Work out the finished part from the listing and answer in its coordinate system (mm). A direction names the side the tool comes from. Coordinates: 2 decimals unless noted, no trailing zeros. Loops run counter-clockwise (first coordinate to the right, second up) from the corner with the lowest first, then second, coordinate; pieces in that order, holes last. Notation, with made-up numbers: (-36, 38) - (-31, 38) arc R17 ccw to (-31, 52) - close; hole circle Ø11 at (75.5, -27.5). An arc over 180 degrees is marked (long way). Write each question's results on one line, items separated by ' | '. Start each with the question number.
1. A cutting plane is placed at C-C on z = -22. Determine the outline of the cut face in (x, y), then the cut area to 3 significant figures.
2. A cutting plane is placed at A-A on y = 20. Determine the outline of the cut face in (x, z), then the cut area to 3 significant figures.
3. Determine the mould class of faces 5 (the flat face through (32, 14, 110)), 6 (the flat face through (32, 13, -112)), 7 (the flat face through (100, 9, -111)), 8 (the flat face through (10, 1, -2)) for opening direction Z: released by +Z, released by -Z, zero draft, split by the parting line, or undercut.
4. Each of these flat-tipped pins is pushed along its axis until it touches: P1, Ø10, axis at y = 9, z = -52, coming from the +X side; P2, Ø0.6, axis at y = 13.5, z = -111, coming from the +X side; P3, Ø1, axis at x = 11, z = 111, coming from the +Y side; P4, Ø1.5, axis at x = 17.5, y = 24.5, coming from the +Z side. Where does it stop, or does it pass through?
5. Which of the six approach directions +Z, -Z, +X, -X, +Y, -Y give full straight-line access (tool end or side, diameter ignored) to faces 1 (the flat face through (-35, 9, -111)), 2 (the flat face through (32, 14, -110)), 3 (the flat face through (100, 8, 111)), 4 (the flat face through (-35, 9, 111))?
6. Find the intervals of material crossed by line 1 along Z through (x, y) = (-31.5, 7.5); line 2 along Y through (x, z) = (-22, -84); line 3 along X through (y, z) = (13, -18.5), in increasing order. Write a range as [from, to].
7. A cutting plane is placed at B-B on x = 15. Determine the outline of the cut face in (y, z).
from build123d import *

# Parameters (mm, degrees)
SKETCH1_W                    = 200
SKETCH1_H                    = 224
BOSS_EXTRUDE1_DEPTH          = 1
SKETCH41_W                   = 65
SKETCH41_H                   = 15
CUT_EXTRUDE2_DEPTH           = 40
EDGE_FLANGE1_STRIP_W         = 12
EDGE_FLANGE1_STRIP_H         = 2
EDGE_FLANGE1_STRIP_CUT_DEPTH = 135
EDGE_FLANGE1_DEPTH           = 135
SKETCH53_W                   = 194
SKETCH53_H                   = 2
BOSS_EXTRUDE2_DEPTH          = 20
CUT_EXTRUDE3_DEPTH           = 20
EDGE_FLANGE3_STRIP_W         = 12
EDGE_FLANGE3_STRIP_H         = 2
EDGE_FLANGE3_STRIP_CUT_DEPTH = 194
EDGE_FLANGE3_DEPTH           = 194
SKETCH58_W                   = 2
SKETCH58_H                   = 36
BOSS_EXTRUDE3_DEPTH          = 14
CUT_EXTRUDE4_DEPTH           = 10


# Sheet-metal steps are written as plain solids
with BuildPart() as part:
    # Sketch1 → Boss-Extrude1 (new, symmetric)
    with BuildSketch(Plane(origin=(0, 0, 0), x_dir=(1, 0, 0), z_dir=(0, 1, 0))):
        Rectangle(SKETCH1_W, SKETCH1_H)
    extrude(amount=BOSS_EXTRUDE1_DEPTH, both=True)

    # Sketch41 → Cut-Extrude2 (cut)
    with BuildSketch(Plane(origin=(0, 1, 0), x_dir=(1, 0, 0), z_dir=(0, 1, 0))):
        with Locations((-67.5, -104.5)):
            Rectangle(SKETCH41_W, SKETCH41_H)
        with Locations((-67.5, 104.5)):
            Rectangle(SKETCH41_W, SKETCH41_H)
    extrude(amount=-CUT_EXTRUDE2_DEPTH, mode=Mode.SUBTRACT)

    # Edge-Flange1 strip (across the edge) → Edge-Flange1 strip cut (cut)
    with BuildSketch(Plane(origin=(-35, 1, 112), x_dir=(0, 0, -1), z_dir=(1, 0, 0))):
        with Locations((-2, -1)):
            Rectangle(EDGE_FLANGE1_STRIP_W, EDGE_FLANGE1_STRIP_H)
    edge_flange1_strip_cut = extrude(amount=EDGE_FLANGE1_STRIP_CUT_DEPTH, mode=Mode.SUBTRACT)

    # Edge-Flange1 section (across the edge) → Edge-Flange1 (add)
    with BuildSketch(Plane(origin=(-35, 1, 112), x_dir=(0, 0, -1), z_dir=(1, 0, 0))):
        with BuildLine():
            Line((0, 2), (0, 23))
            Line((0, 23), (2, 23))
            Line((2, 23), (2, 2))
            ThreePointArc((2, 2), (2.585786438, 0.585786438), (4, 0))
            Line((4, 0), (4, -2))
            ThreePointArc((4, -2), (1.171572875, -0.828427125), (0, 2))
        make_face()
    edge_flange1 = extrude(amount=EDGE_FLANGE1_DEPTH)

    # Mirror1: Edge-Flange1 strip cut, Edge-Flange1 across plane
    add(edge_flange1_strip_cut.mirror(Plane.XY), mode=Mode.SUBTRACT)
    add(edge_flange1.mirror(Plane.XY))

    # Sketch53 → Boss-Extrude2 (add)
    with BuildSketch(Plane(origin=(100, 0, 0), x_dir=(0, 0, -1), z_dir=(1, 0, 0))):
        Rectangle(SKETCH53_W, SKETCH53_H)
    extrude(amount=BOSS_EXTRUDE2_DEPTH)

    # Sketch54 → Cut-Extrude3 (cut)
    with BuildSketch(Plane(origin=(0, 0, 110), x_dir=(-1, 0, 0), z_dir=(0, 0, -1))):
        with BuildLine():
            Line((-94.5, 8.506539698), (-94.5, 15.506539698))
            ThreePointArc((-94.5, 15.506539698), (-93, 17.006539698), (-91.5, 15.506539698))
            Line((-91.5, 15.506539698), (-91.5, 8.506539698))
            ThreePointArc((-91.5, 8.506539698), (-93, 7.006539698), (-94.5, 8.506539698))
        make_face()
        with BuildLine():
            Line((-85.5, 8.506539698), (-85.5, 15.506539698))
            ThreePointArc((-85.5, 15.506539698), (-84, 17.006539698), (-82.5, 15.506539698))
            Line((-82.5, 15.506539698), (-82.5, 8.506539698))
            ThreePointArc((-82.5, 8.506539698), (-84, 7.006539698), (-85.5, 8.506539698))
        make_face()
        with BuildLine():
            Line((-76.5, 8.506539698), (-76.5, 15.506539698))
            ThreePointArc((-76.5, 15.506539698), (-75, 17.006539698), (-73.5, 15.506539698))
            Line((-73.5, 15.506539698), (-73.5, 8.506539698))
            ThreePointArc((-73.5, 8.506539698), (-75, 7.006539698), (-76.5, 8.506539698))
        make_face()
        with BuildLine():
            Line((14.5, 8.506539698), (14.5, 15.506539698))
            ThreePointArc((14.5, 15.506539698), (16, 17.006539698), (17.5, 15.506539698))
            Line((17.5, 15.506539698), (17.5, 8.506539698))
            ThreePointArc((17.5, 8.506539698), (16, 7.006539698), (14.5, 8.506539698))
        make_face()
        with BuildLine():
            Line((5.5, 8.506539698), (5.5, 15.506539698))
            ThreePointArc((5.5, 15.506539698), (7, 17.006539698), (8.5, 15.506539698))
            Line((8.5, 15.506539698), (8.5, 8.506539698))
            ThreePointArc((8.5, 8.506539698), (7, 7.006539698), (5.5, 8.506539698))
        make_face()
        with BuildLine():
            Line((23.5, 8.506539698), (23.5, 15.506539698))
            ThreePointArc((23.5, 15.506539698), (25, 17.006539698), (26.5, 15.506539698))
            Line((26.5, 15.506539698), (26.5, 8.506539698))
            ThreePointArc((26.5, 8.506539698), (25, 7.006539698), (23.5, 8.506539698))
        make_face()
    cut_extrude3 = extrude(amount=-CUT_EXTRUDE3_DEPTH, mode=Mode.SUBTRACT)

    # Edge-Flange3 strip (across the edge) → Edge-Flange3 strip cut (cut)
    with BuildSketch(Plane(origin=(-100, 1, -97), x_dir=(1, 0, 0), z_dir=(0, 0, 1))):
        with Locations((-2, -1)):
            Rectangle(EDGE_FLANGE3_STRIP_W, EDGE_FLANGE3_STRIP_H)
    extrude(amount=EDGE_FLANGE3_STRIP_CUT_DEPTH, mode=Mode.SUBTRACT)

    # Edge-Flange3 section (across the edge) → Edge-Flange3 (add)
    with BuildSketch(Plane(origin=(-100, 1, -97), x_dir=(1, 0, 0), z_dir=(0, 0, 1))):
        with BuildLine():
            Line((0, 2), (0, 38))
            Line((0, 38), (2, 38))
            Line((2, 38), (2, 2))
            ThreePointArc((2, 2), (2.585786438, 0.585786438), (4, 0))
            Line((4, 0), (4, -2))
            ThreePointArc((4, -2), (1.171572875, -0.828427125), (0, 2))
        make_face()
    extrude(amount=EDGE_FLANGE3_DEPTH)

    # Sketch58 → Boss-Extrude3 (add)
    with BuildSketch(Plane.XY.offset(97)):
        with Locations((-99, 21)):
            Rectangle(SKETCH58_W, SKETCH58_H)
    boss_extrude3 = extrude(amount=BOSS_EXTRUDE3_DEPTH)

    # Mirror2: Cut-Extrude3, Boss-Extrude3 across plane
    add(cut_extrude3.mirror(Plane.XY), mode=Mode.SUBTRACT)
    add(boss_extrude3.mirror(Plane.XY))

    # Sketch59 → Cut-Extrude4 (cut)
    with BuildSketch(Plane(origin=(0, 1, 0), x_dir=(1, 0, 0), z_dir=(0, 1, 0))):
        with BuildLine():
            Line((111, -90), (111, -70))
            ThreePointArc((111, -70), (112.5, -68.5), (114, -70))
            Line((114, -70), (114, -90))
            ThreePointArc((114, -90), (112.5, -91.5), (111, -90))
        make_face()
        with BuildLine():
            Line((111, -10), (111, 10))
            ThreePointArc((111, 10), (112.5, 11.5), (114, 10))
            Line((114, 10), (114, -10))
            ThreePointArc((114, -10), (112.5, -11.5), (111, -10))
        make_face()
        with BuildLine():
            Line((111, 90), (111, 70))
            ThreePointArc((111, 70), (112.5, 68.5), (114, 70))
            Line((114, 70), (114, 90))
            ThreePointArc((114, 90), (112.5, 91.5), (111, 90))
        make_face()
    extrude(amount=-CUT_EXTRUDE4_DEPTH, mode=Mode.SUBTRACT)


solid = part.part
Values:
1) outline: (-100, 3) arc R4 ccw to (-96, -1) - (120, -1) - (120, 1) - (-96, 1) arc R2 cw to (-98, 3) - (-98, 39) - (-100, 39) - close | area: 513 mm^2
2) outline: (-100, -111) - (-98, -111) - (-98, 111) - (-100, 111) - close; (-35, -112) - (100, -112) - (100, -110) - (-35, -110) - close; (-35, 110) - (100, 110) - (100, 112) - (-35, 112) - close | area: 984 mm^2
3) face 5: undercut | face 6: released by -Z | face 7: zero draft | face 8: undercut
4) P1: x = -98 | P2: x = 100 | P3: y = 24 | P4: z = 112
5) face 1: -Z, +Y, -Y | face 2: +X, +Y | face 3: +Z, +X, +Y, -Y | face 4: +Z, +Y, -Y
6) line 1: [-112, -110], [110, 112] | line 2: [-1, 1] | line 3: [-100, -98]
7) outline: (-1, -108) arc R4 ccw to (3, -112) - (24, -112) - (24, -110) - (3, -110) arc R2 cw to (1, -108) - (1, 108) arc R2 cw to (3, 110) - (24, 110) - (24, 112) - (3, 112) arc R4 ccw to (-1, 108) - close
